Autodesk Inventor part; units mm, degrees
ref_plane "YZ Plane" through (0, 0, 0) normal (1, 0, 0) x (0, 1, 0)
ref_plane "XZ Plane" through (0, 0, 0) normal (0, 1, 0) x (-1, 0, 0)
ref_plane "XY Plane" through (0, 0, 0) normal (0, 0, 1) x (1, 0, 0)
sketch "Esboço1" plane through (0, 0, 0) normal (0, 0, 1) x (1, 0, 0)
  line L0 (-18.5, 0) -> (18.5, 0) construction
  line L1 (-24, 0) -> (24, 0) construction
  line L2 (-20.8784, 4.9592) -> (-5.7013, 12.238)
  line L3 (20.8784, 4.9592) -> (5.8378, 12.1725)
  line L4 (-20.8784, -4.9592) -> (-5.5742, -12.299)
  line L5 (5.8378, -12.1725) -> (20.8784, -4.9592)
  arc A0 (20.8784, -4.9592) -> (20.8784, 4.9592) centre (18.5, 0) ccw
  arc A1 (-5.8378, -12.1725) -> (5.8378, -12.1725) centre (0, 0) ccw
  arc A2 (5.8378, 12.1725) -> (-5.8378, 12.1725) centre (0, 0) ccw
  arc A3 (-20.8784, 4.9592) -> (-20.8784, -4.9592) centre (-18.5, 0) ccw
  dimension "d1" = 37
  dimension "d2" = 48
extrude "Extrusão1" add sketch "Esboço1" along normal blind 4
sketch "Esboço2" plane through (0, 0, 4) normal (0, 0, 1) x (1, 0, 0)
  circle A0 centre (0, 0) radius 13.5
  circle A1 centre (0, 0) radius 14.5
  dimension "d5" = 27
  dimension "d6" = 29
extrude "Extrusão2" cut sketch "Esboço2" against normal blind 1
sketch "Esboço3" plane through (0, 0, 4) normal (0, 0, 1) x (1, 0, 0)
  circle A0 centre (0, 0) radius 13.5
  dimension "d9" = 27
extrude "Extrusão3" add sketch "Esboço3" along normal blind 4.5
sketch "Esboço4" plane through (0, 0, 8.5) normal (0, 0, 1) x (1, 0, 0)
  circle A0 centre (0, 0) radius 11.5
  dimension "d12" = 23
extrude "Extrusão4" cut sketch "Esboço4" against normal blind 1.5
sketch "Esboço5" plane through (0, 0, 0) normal (0, 0, -1) x (-1, 0, 0)
  circle A0 centre (0, 0) radius 11.5
  dimension "d15" = 23
extrude "Extrusão5" cut sketch "Esboço5" against normal blind 1.5
sketch "Esboço6" plane through (0, 0, 8.5) normal (0, 0, 1) x (1, 0, 0)
  circle A0 centre (0, 0) radius 13
  circle A1 centre (0, 0) radius 13.25
  dimension "d18" = 26
  dimension "d19" = 26.5
extrude "Extrusão6" cut sketch "Esboço6" against normal blind 0.2
sketch "Esboço8" plane through (0, 0, 0) normal (0, 0, -1) x (-1, 0, 0)
  circle A0 centre (0, 0) radius 13
  circle A1 centre (0, 0) radius 13.25
  dimension "d22" = 26
  dimension "d23" = 26.5
extrude "Extrusão7" cut sketch "Esboço8" against normal blind 0.2
sketch "Esboço9" plane through (0, 0, 7) normal (0, 0, 1) x (1, 0, 0)
  circle A0 centre (0, 0) radius 6
  dimension "d26" = 12
extrude "Extrusão8" add sketch "Esboço9" along normal blind 4
sketch "Esboço10" plane through (0, 0, 1.5) normal (0, 0, -1) x (-1, 0, 0)
  circle A0 centre (0, 0) radius 6
  dimension "d29" = 12
extrude "Extrusão9" add sketch "Esboço10" along normal blind 1.5
sketch "Esboço11" plane through (0, 0, 11) normal (0, 0, 1) x (1, 0, 0)
  circle A0 centre (0, 0) radius 2.3758
hole "Furo1" at (0, 0, 11) direction (0, 0, -1) diameter 8 end through all
sketch "Esboço12" plane through (0, 0, 0) normal (0, 0, -1) x (-1, 0, 0)
  line L0 (18.5, 0) -> (-18.5, 0) construction
  circle A0 centre (18.5, 0) radius 0.9755 construction
  circle A1 centre (-18.5, 0) radius 0.8896 construction
  point P0 (0, 0)
  point P1 (0, 0)
  dimension "d39" = 37
hole "Furo2" at (-18.5, 0, 0) at (18.5, 0, 0) direction (0, 0, 1) diameter 4.8 end through all
properties part number "KFL08"
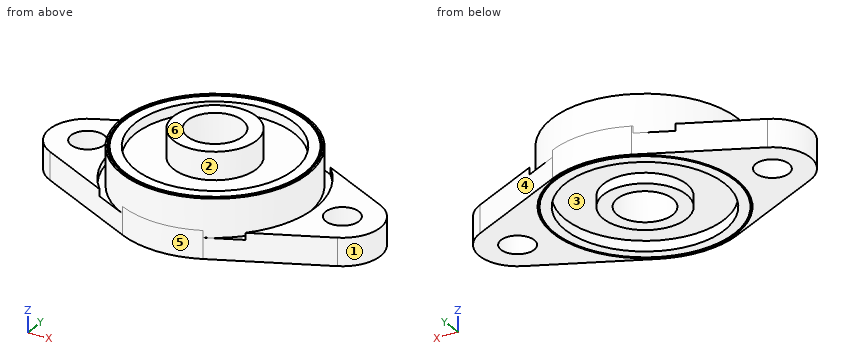
The model under review builds one solid part; all positions refer to its coordinate system, in mm. Face numbers are marked on the shaded views. A direction names the side the tool comes from. Round coordinates to 2 decimals unless told otherwise and drop trailing zeros. Loops run counter-clockwise (first coordinate to the right, second up) from the corner with the lowest first, then second, coordinate; pieces in that order, holes last. Notation, with made-up numbers: M 73.5,74.5 L 97.5,74.5 A27 cw 97.5,107.5 Z; hole C 84,-14 d2. An arc over 180 degrees is marked long. Answer as CSV lines item,"result". Start each with the question number.
Item 1: Mouldability with a two-part tool opening along Y and no side actions: class the marked faces 3, 4, 5 and 6 as released by +Y, released by -Y, zero draft, split by the parting line, or undercut.
Item 2: Wall thickness on line 1 (Y direction, x = 0, z = 7.9); line 2 (X direction, y = 5, z = 0.5); line 3 (Y direction, x = -9.5, z = 1.25): over which ranges is each line inside the solid? List them lowest first. Write a range as [from, to].
Item 3: Consider section B-B (y = 0). State how many separate pieces and enclosed holes the cut face has, then the cut area to 3 significant figures.
Item 4: Consider section A-A (z = 2). Write out the cut boundary in (x, y).
Item 5: Consider section C-C (x = 14). Write out the cut boundary in (y, z), then the cut area to 3 significant figures.
Item 6: Insertion check: P1, Ø14, axis at x = 0, y = 0, coming from the -Z side; P2, Ø5, axis at y = 5.5, z = 7, coming from the +X side; P3, Ø7.5, axis at x = -18.5, y = 0, coming from the +Z side; P4, Ø2, axis at x = -9.5, y = -3, coming from the +Z side. Each pin has a flat end and moves straight along its axis. Give the tip position at first contact, or say it passes through.
Item 7: Consider section D-D (z = 6.5). Write out the cut boundary in (x, y).
Item 8: For the marked faces 1 and 2, list the 3-axis set-ups (+Z, -Z, +X, -X, +Y, -Y) from which the entire face can be reached by the end or side of a thin tool; tool diameter is ignored.
Answer:
1,face 3,"undercut"
1,face 4,"released by +Y"
1,face 5,"released by -Y"
1,face 6,"zero draft"
2,line 1,"y = [-13.5, -11.5], [-6, -4], [4, 6], [11.5, 13.5]"
2,line 2,"x = [-20.79, -10.36], [-3.32, 3.32], [10.36, 20.79]"
2,line 3,"y = [-10.42, -6.48], [6.48, 10.42]"
3,separate pieces,"4"
3,enclosed holes,"0"
3,area,"182 mm^2"
4,outline,"M -20.88,-4.96 L -5.84,-12.17 A13.5 ccw 5.84,-12.17 L 20.88,-4.96 A5.5 ccw 20.88,4.96 L 5.84,12.17 A13.5 ccw -5.7,12.24 L -20.88,4.96 A5.5 ccw Z; hole C -18.5,0 d4.8; hole C 0,0 d8; hole C 18.5,0 d4.8"
5,outline,"M -8.26,0 L 8.26,0 L 8.26,4 L 3.77,4 L 3.77,3 L -3.77,3 L -3.77,4 L -8.26,4 Z"
5,area,"58.5 mm^2"
6,P1,"stops at z = 0"
6,P2,"stops at x = 13.16"
6,P3,"stops at z = 4"
6,P4,"stops at z = 7"
7,outline,"C 0,0 d27; hole C 0,0 d8"
8,face 1,"+Z, -Z, +X"
8,face 2,"+Z"
